Verification items for the finished model (mm, model axes). A direction names the side the tool comes from. Give positions to 0.01 mm unless a question says otherwise; leave off trailing zeros. Loops run counter-clockwise (first coordinate to the right, second up) from the corner with the lowest first, then second, coordinate; pieces in that order, holes last. Notation, with made-up numbers: (-31.75, 19) - (17.25, 19) arc R16 cw to (17.25, 32) - close; hole circle Ø11 at (2.5, 74). An arc over 180 degrees is marked (long way). Answer in a Markdown table with one row per item.
```python
from build123d import *

# Parameters (mm, degrees)
SKETCH1_W           = 15
SKETCH1_H           = 30
SKETCH1_R           = 1.5
BOSS_EXTRUDE1_DEPTH = 2
SKETCH2_R           = 1.5
BOSS_EXTRUDE2_DEPTH = 2.5


with BuildPart() as part:
    # Sketch1 → Boss-Extrude1 (new body)
    with BuildSketch(Plane.XY):
        Rectangle(SKETCH1_W, SKETCH1_H)
        with Locations((0, 10)):
            Circle(SKETCH1_R, mode=Mode.SUBTRACT)
        with Locations((0, -10)):
            Circle(SKETCH1_R, mode=Mode.SUBTRACT)
    extrude(amount=BOSS_EXTRUDE1_DEPTH)

    # Sketch2 → Boss-Extrude2 (add, symmetric)
    with BuildSketch(Plane(origin=(0, 0, 0), x_dir=(1, 0, 0), z_dir=(0, 1, 0))):
        with BuildLine():
            Line((-3, 0), (3, 0))
            Line((3, 0), (3, 10))
            ThreePointArc((3, 10), (2.267766953, 11.767766953), (0.5, 12.5))
            Line((0.5, 12.5), (-15.5, 12.5))
            ThreePointArc((-15.5, 12.5), (-19.5, 8.5), (-15.5, 4.5))
            Line((-15.5, 4.5), (-7.5, 4.5))
            ThreePointArc((-7.5, 4.5), (-4.318019485, 3.181980515), (-3, 0))
        make_face()
        with Locations(Location((-15.5, 8.5, 0), (0, 0, 270))):
            Circle(SKETCH2_R, mode=Mode.SUBTRACT)
    extrude(amount=BOSS_EXTRUDE2_DEPTH, both=True)


solid = part.part
```
Q1. Draft check along X on faces 5 (the face through (0, 0, 2)), 6 (the face through (7.5, 0, 1)), 7 (the face through (-15.43, -0.04, -10)). Enter one of: +X half, -X half, draft (parallel to the pull), parting line (faces both ways), or undercut.
Completed:
| item | result |
|---|---|
| face 5 | draft |
| face 6 | +X half |
| face 7 | undercut |
Q2. Tool access check on faces 1 (the face through (-6, 2.5, -8)), 2 (the face through (-4.353, 0.035, -3.217)), 3 (the face through (3, 0, -5)), 4 (the face through (-12, 0, -4.5)). Record the directions out of +Z, -Z, +X, -X, +Y, -Y that give a thin tool (end or side, any length) a straight path to the whole face; none if there is none.
Completed:
| item | result |
|---|---|
| face 1 | -Z, +X, -X, +Y |
| face 2 | -X, +Y, -Y |
| face 3 | -Z, +X, +Y, -Y |
| face 4 | +Z, -X, +Y, -Y |
Q3. Sectioned sample at A-A (y = -10). Record the cut outline in (x, z).
Completed:
| item | result |
|---|---|
| outline | (-7.5, 0) - (-1.5, 0) - (-1.5, 2) - (-7.5, 2) - close; (1.5, 0) - (7.5, 0) - (7.5, 2) - (1.5, 2) - close |
Q4. Thickness scan on line 1 (Y direction, x = 0, z = 1.45); line 2 (Z direction, x = 6.25, y = 8); line 3 (Y direction, x = -10, z = -8). Record the ranges inside material, lowest first.
Completed:
| item | result |
|---|---|
| line 1 | -15 to -11.5, -8.5 to 8.5, 11.5 to 15 |
| line 2 | 0 to 2 |
| line 3 | -2.5 to 2.5 |
Q5. Go/stop test with flat-tipped pins: P1, Ø4, axis at y = 1, z = -7, coming from the +X side; P2, Ø3.5, axis at x = -15.5, z = -8.5, coming from the +Y side; P3, Ø1.5, axis at x = 4.5, y = 8.5, coming from the -Z side. Record where each tip stops, or that it passes through.
Completed:
| item | result |
|---|---|
| P1 | x = 3 |
| P2 | y = 2.5 |
| P3 | z = 0 |
Q6. Sectioned sample at B-B (x = 0). Record the cut outline in (y, z), and give its area (4 significant figures).
Completed:
| item | result |
|---|---|
| outline | (-15, 0) - (-11.5, 0) - (-11.5, 2) - (-15, 2) - close; (-8.5, 0) - (-2.5, 0) - (-2.5, -12.5) - (2.5, -12.5) - (2.5, 0) - (8.5, 0) - (8.5, 2) - (-8.5, 2) - close; (11.5, 0) - (15, 0) - (15, 2) - (11.5, 2) - close |
| area | 110.5 mm^2 |
Q7. Sectioned sample at D-D (y = -1). Record the cut outline in (x, z), and give its area (3 significant figures).
Completed:
| item | result |
|---|---|
| outline | (-15.5, -12.5) - (0.5, -12.5) arc R2.5 ccw to (3, -10) - (3, 0) - (7.5, 0) - (7.5, 2) - (-7.5, 2) - (-7.5, 0) - (-3, 0) arc R4.5 cw to (-7.5, -4.5) - (-15.5, -4.5) arc R4 ccw to start; hole circle Ø3 at (-15.5, -8.5) |
| area | 226 mm^2 |
Q8. Sectioned sample at C-C (z = -8.5). Record the cut outline in (x, y), and give its area (3 significant figures).
Completed:
| item | result |
|---|---|
| outline | (-19.5, -2.5) - (-17, -2.5) - (-17, 2.5) - (-19.5, 2.5) - close; (-14, -2.5) - (3, -2.5) - (3, 2.5) - (-14, 2.5) - close |
| area | 97.5 mm^2 |
